Could you check a few things on this drawing? It's one solid part, dimensions in mm from its lowest x, y, z. A direction names the side the tool comes from. Give positions to 0.01 mm unless a question says otherwise; leave off trailing zeros. Order: outer loops, then holes, each group sorted by start corner. A loop starts at its lowest first (then second) coordinate and runs counter-clockwise, first axis right, second up.
(1) If I drill on probe 1 along Y at (x, z) = (7, 51); probe 2 along Y at (x, z) = (52, 34.5); probe 3 along X at (y, z) = (23.5, 58), over which ranges is the centre line in solid material (lowest first)?
(2) Will these pins go through, and if not, where does the flat tip stop? pin 1 (12 mm diameter, centred on y = 45.5, z = 37.5, fed in from +X); pin 2 (19 mm diameter, centred on x = 62.5, z = 45.5, fed in from -Y); pin 3 (13 mm diameter, centred on y = 20, z = 51, fed in from -X); pin 4 (12 mm diameter, centred on x = 30, z = 50.5, fed in from -Y).
(3) Imagine slicing it at B-B, the plane z = 37.5. Write out the boundary of the cut face in (x, y), then the cut area to 3 significant figures.
(4) Imagine slicing it at C-C, the plane y = 58.5. Write out the boundary of the cut face in (x, z), then the cut area to 3 significant figures.
(5) Imagine slicing it at D-D, the plane z = 6. Write out the boundary of the cut face in (x, y), then the cut area to 3 significant figures.
(6) On a 3-axis mill with a long thin cutter (end or side, diameter ignored), from which of +Z, -Z, +X, -X, +Y, -Y can I reach the whole of each face in a straight line? I mean the marked faces 5 and 6. Say none if no direction works.
(7) Imagine slicing it at A-A, the plane y = 20. Write out the boundary of the cut face in (x, z), then the cut area to 3 significant figures.
(8) If we mould it in two halves opening along X, with no side actions, what happens to the marked faces 1, 2, 3 and 4? For each: released by +X, released by -X, zero draft, split by the parting line, or undercut.
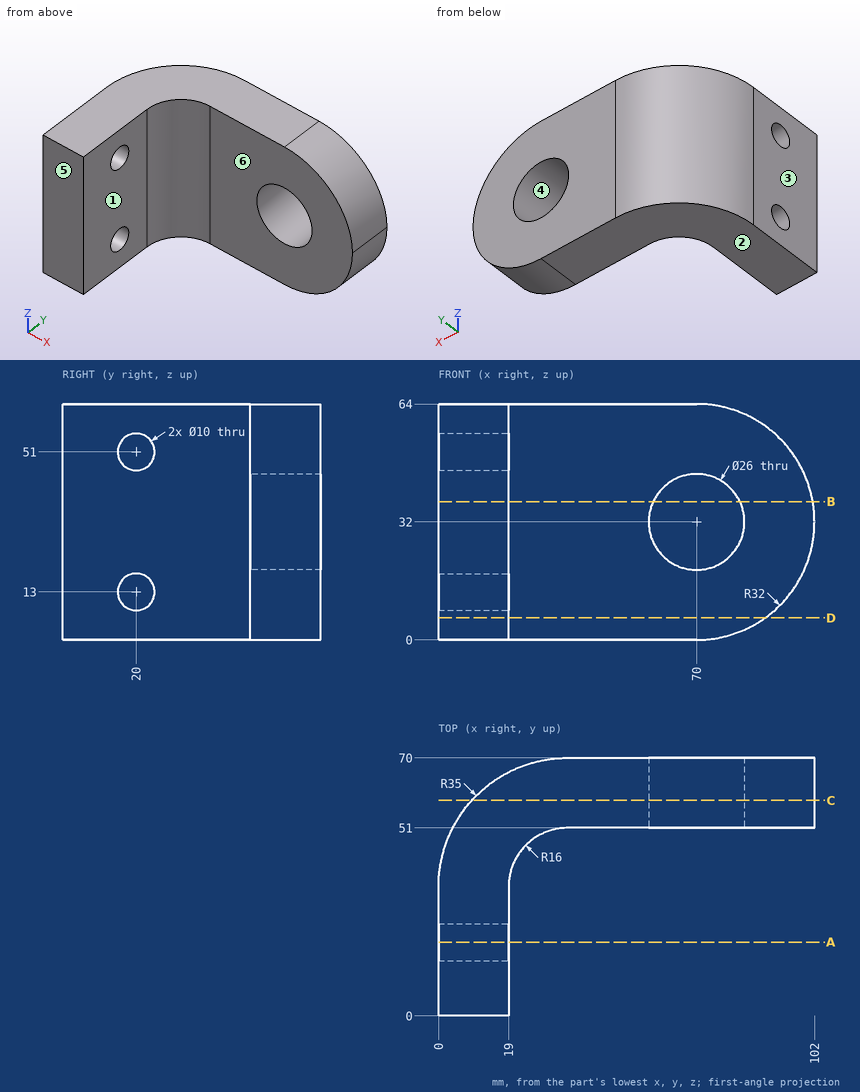
Answer block:
1. probe 1: y = 0 to 15, 25 to 56
1. probe 2: y = 51 to 70
1. probe 3: x = 0 to 19
2. pin 1: stops at x = 101.85
2. pin 2: stops at y = 51
2. pin 3: stops at x = 0
2. pin 4: stops at y = 46.62
3. outline: (0, 0) - (19, 0) - (19, 35) arc R16 cw to (35, 51) - (58.22, 51) - (58.22, 70) - (35, 70) arc R35 ccw to (0, 35) - close; (81.78, 51) - (101.52, 51) - (101.52, 70) - (81.78, 70) - close
3. area: 2,240 mm2
4. outline: (9.06, 0) - (70, 0) arc R32 ccw to (70, 64) - (9.06, 64) - close; hole circle Ø26 at (70, 32)
4. area: 4,980 mm2
5. outline: (0, 0) - (19, 0) - (19, 35) arc R16 cw to (35, 51) - (88.65, 51) - (88.65, 70) - (35, 70) arc R35 ccw to (0, 35) - close
5. area: 2,450 mm2
6. face 5: +Z, -Z, +X, -X, -Y
6. face 6: +Z, -Z, +X, -Y
7. outline: (0, 0) - (19, 0) - (19, 8) - (0, 8) - close; (0, 18) - (19, 18) - (19, 46) - (0, 46) - close; (0, 56) - (19, 56) - (19, 64) - (0, 64) - close
7. area: 836 mm2
8. face 1: released by +X
8. face 2: zero draft
8. face 3: released by -X
8. face 4: undercut
